Build history of the part. All positions in model axes, mm. Face numbers are marked on the shaded views. A direction names the side the tool comes from. Give positions to 0.01 mm unless a question says otherwise; leave off trailing zeros. Write each loop counter-clockwise with the first axis right and the second up, starting at its lowest first coordinate (ties: lowest second). Pieces come first, ordered by that corner, then holes. Notation, with made-up numbers: M -23,48.5 L -10,48.5 A27 ccw -10,85.5 Z; hole C -1.5,18.25 d4. An arc over 180 degrees is marked long. One line per item, written item: value. Start each with the question number.
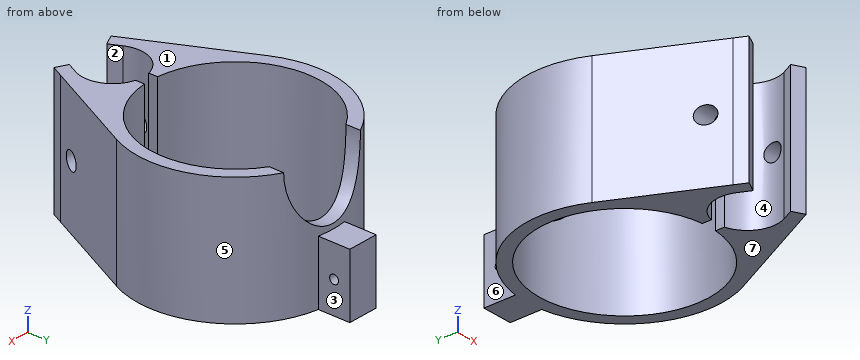
from build123d import *

# Parameters (mm, degrees)
F0_R      = 12
F0_R_2    = 33.5
F1_DEPTH  = 50
F4_DEPTH  = 25
F5_W      = 12
F5_H      = 25
F6_DEPTH  = 1
F7_DEPTH  = 12
F8_R      = 3.429
F9_DEPTH  = 30
F10_R     = 1.75
F11_DEPTH = 25
F12_W     = 6
F12_H     = 8.7619052733
F13_DEPTH = 55
F15_DEPTH = 52
F17_DEPTH = 50


with BuildPart() as f1:
    # F0 (on Top) → F1 (new body)
    with BuildSketch(Plane.XY):
        with BuildLine():
            ThreePointArc((34.510392045, 31.4329896907), (0, 87), (-34.510392045, 31.4329896907))
            Line((-34.510392045, 31.4329896907), (-15.238354929, -7.5360824742))
            ThreePointArc((-15.238354929, -7.5360824742), (0, -17), (15.238354929, -7.5360824742))
            Line((15.238354929, -7.5360824742), (34.510392045, 31.4329896907))
        make_face()
        Circle(F0_R, mode=Mode.SUBTRACT)
        with Locations((0, 48.5)):
            Circle(F0_R_2, mode=Mode.SUBTRACT)
    extrude(amount=F1_DEPTH)

    # F3 (on offset) → F4 (cut)
    with BuildSketch(Plane.XZ.offset(-87)):
        with BuildLine():
            add(Edge.make_bspline(
                [(17.5, 50), (17.5, 73), (0, 73), (-17.5, 73), (-17.5, 50)],
                knots=[1.5707963268, 1.5707963268, 1.5707963268, 3.1415926536, 3.1415926536, 4.7123889804, 4.7123889804, 4.7123889804], degree=2, weights=[1, 0.7071067812, 1, 0.7071067812, 1]))
            Line((-17.5, 50), (17.5, 50))
        make_face()
        with BuildLine():
            Line((17.5, 50), (-17.5, 50))
            add(Edge.make_bspline(
                [(-17.5, 50), (-17.5, 27), (0, 27)],
                knots=[4.7123889804, 4.7123889804, 4.7123889804, 6.2831853072, 6.2831853072, 6.2831853072], degree=2, weights=[1, 0.7071067812, 1]))
            add(Edge.make_bspline(
                [(0, 27), (17.5, 27), (17.5, 50)],
                knots=[0, 0, 0, 1.5707963268, 1.5707963268, 1.5707963268], degree=2, weights=[1, 0.7071067812, 1]))
        make_face()
    extrude(amount=F4_DEPTH, mode=Mode.SUBTRACT)

    # F5 (on offset) → F6 (join)
    with BuildSketch(Plane.XZ.offset(-87)):
        with Locations((0, 12.5)):
            Rectangle(F5_W, F5_H)
    extrude(amount=F6_DEPTH)

    # F5 (on offset) → F7 (join)
    with BuildSketch(Plane.XZ.offset(-87)):
        with Locations((0, 12.5)):
            Rectangle(F5_W, F5_H)
    extrude(amount=-F7_DEPTH)

    # F8 (on Right) → F9 (cut, symmetric)
    with BuildSketch(Plane.YZ):
        with Locations((0, 25)):
            Circle(F8_R)
    extrude(amount=F9_DEPTH, both=True, mode=Mode.SUBTRACT)

    # F10 (on face) → F11 (cut)
    with BuildSketch(Plane(origin=(-6, 0, 0), x_dir=(0, -1, 0), z_dir=(-1, 0, 0))):
        with Locations((-92.7647968698, 12.5)):
            Circle(F10_R)
    extrude(amount=-F11_DEPTH, mode=Mode.SUBTRACT)

    # F12 (on face) → F13 (cut)
    with BuildSketch(Plane.XY.offset(50)):
        with Locations((0, 13.4115335532)):
            Rectangle(F12_W, F12_H)
    extrude(amount=-F13_DEPTH, mode=Mode.SUBTRACT)

    # F14 (on face) → F15 (cut)
    with BuildSketch(Plane.XY.offset(50)):
        with BuildLine():
            ThreePointArc((10.7564858322, -5.3195876289), (0, -12), (-10.7564858322, -5.3195876289))
            Line((-10.7564858322, -5.3195876289), (-15.238354929, -7.5360824742))
            ThreePointArc((-15.238354929, -7.5360824742), (0, -17), (15.238354929, -7.5360824742))
            Line((15.238354929, -7.5360824742), (10.7564858322, -5.3195876289))
        make_face()
    extrude(amount=-F15_DEPTH, mode=Mode.SUBTRACT)

    # F16 (on Top) → F17 (join)
    with BuildSketch(Plane.XY):
        Polygon((-10.7564858322, -5.3195876289), (-15.238354929, -7.5360824742), (-13.0218600836, -12.017951571), (-8.5399909869, -9.8014567256), align=None)
        Polygon((13.0218600836, -12.017951571), (15.238354929, -7.5360824742), (10.7564858322, -5.3195876289), (8.5399909869, -9.8014567256), align=None)
    extrude(amount=F17_DEPTH)


solid = f1.part
1) Tool access for the marked faces 1, 2 and 3: list every direction of +Z, -Z, +X, -X, +Y, -Y with a clear straight run to the whole face (end or side of a thin tool).
2) Band-saw the part on D-D (y = 2). List the corners of the cut face in (x, z), then the cut area to 3 significant figures.
3) Mould opens along X. For the marked faces 4, 5, 6 and 7 say: released by +X, released by -X, zero draft, split by the parting line, or undercut.
4) Probe line 1 along X through (y, z) = (48, 26); line 2 along Z through (x, y) = (14, 0); line 3 along X through (y, z) = (94.5, 17.5). List the from-to ranges inside material, lowest first. Write a range as from..to.
5) Band-saw the part on A-A (y = 48.5). List the corners of the cut face in (x, z).
6) Band-saw the part on C-C (x = -19). List the corners of the cut face in (y, z).
7) Band-saw the part on B-B (z = 12.5). List the corners of the cut face in (x, y), then the cut area to 3 significant figures.
8) Drop flat-ended pins along their axis: P1, Ø10, axis at y = 95.5, z = 13.5, coming from the -X side; P2, Ø3, axis at y = 48, z = 23, coming from the -X side; P3, Ø6, axis at y = 37.5, z = 22.5, coming from the +X side. Give the stop position or say it passes through.
Model answer:
1. face 1: +Z, +X, -X, +Y, -Y
1. face 2: +Z, -Z
1. face 3: +Z, -Z, +X, +Y
2. outline: M -19.95,0 L -11.83,0 L -11.83,22.21 L -19.95,22.21 Z; M -19.95,27.79 L -11.83,27.79 L -11.83,50 L -19.95,50 Z; M 11.83,0 L 19.95,0 L 19.95,22.21 L 11.83,22.21 Z; M 11.83,27.79 L 19.95,27.79 L 19.95,50 L 11.83,50 Z
2. area: 722 mm²
3. face 4: undercut
3. face 5: split by the parting line
3. face 6: released by -X
3. face 7: zero draft
4. line 1: x = -38.5..-33.5, 33.5..38.5
4. line 2: z = 0..21.57, 28.43..50
4. line 3: x = -6..6
5. outline: M -38.5,0 L -33.5,0 L -33.5,50 L -38.5,50 Z; M 33.5,0 L 38.5,0 L 38.5,50 L 33.5,50 Z
6. outline: M 0.07,0 L 20.91,0 L 20.91,50 L 0.07,50 L 0.07,28.43 A3.43 cw 0.07,21.57 Z; M 76.09,0 L 81.99,0 L 81.99,50 L 76.09,50 Z
7. outline: M -34.51,31.43 L -13.02,-12.02 L -8.54,-9.8 L -10.76,-5.32 A12 cw -3,11.62 L -3,15.13 A33.5 cw long 3,15.13 L 3,11.62 A12 cw 10.76,-5.32 L 8.54,-9.8 L 13.02,-12.02 L 34.51,31.43 A38.5 ccw 6,86.53 L 6,91.01 L -6,91.01 L -6,86.53 A38.5 ccw Z; M -6,94.51 L 6,94.51 L 6,99 L -6,99 Z
7. area: 1,740 mm²
8. P1: stops at x = -6
8. P2: stops at x = -38.5
8. P3: stops at x = 37.66
